The figure shows three views and two pictorial views of one solid part (mm, origin at its lowest corner). Answer the questions. Coordinates: 2 decimals unless noted, no trailing zeros. Write each loop counter-clockwise with the first axis right and the second up, starting at its lowest first coordinate (ties: lowest second). Pieces come first, ordered by that corner, then holes. Notation, with made-up numbers: M 65,36.5 L 117,36.5 A4 ccw 117,40.5 Z; hole C 63,53 d10. An arc over 180 degrees is marked long. Use a Markdown table: item, result. Add a question column.
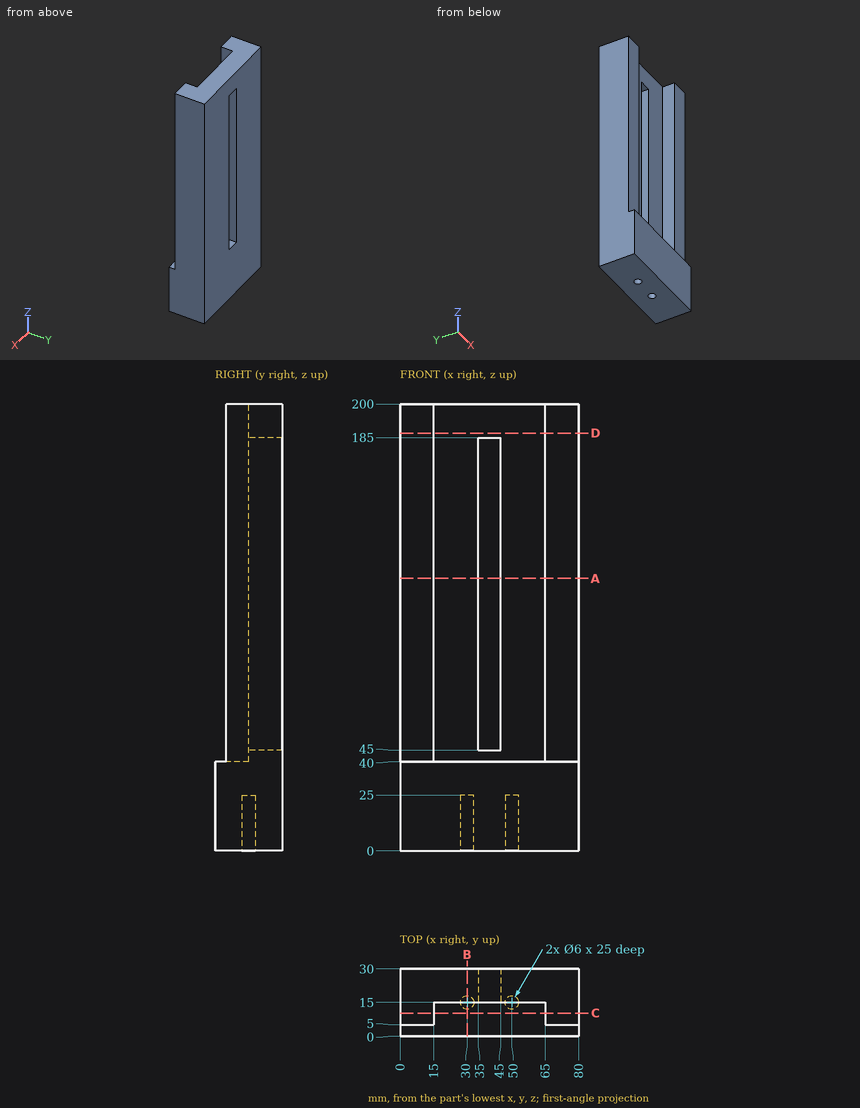
Item 1: Find section A-A on z = 122. Give the vertices of the cut face in (x, y), then the cut area to 3 significant figures.
Item 2: Find section B-B on x = 30. Give the vertices of the cut face in (y, z).
Item 3: Find section D-D on z = 187. Give the vertices of the cut face in (x, y).
Item 4: Consider probe 1 along X at (y, z) = (15, 10.5); probe 2 along Y at (x, z) = (50, 5.5); probe 3 along X at (y, z) = (27.25, 154.5). Determine where each line is inside the solid, lowest interval first.
Item 5: Find section C-C on y = 10.25. Give the vertices of the cut face in (x, z).
Item 6: Each of these flat-tipped pins is pushed along its axis until it touches: pin 1 (7.5 mm diameter, centred on x = 59, y = 10, fed in from +Z); pin 2 (8 mm diameter, centred on x = 46, z = 172.5, fed in from -Y); pin 3 (3 mm diameter, centred on x = 11.5, z = 142.5, fed in from -Y). Where does it stop, or does it pass through?
Geometry says:
| question | item | result |
|---|---|---|
| 1 | outline | M 0,5 L 15,5 L 15,15 L 35,15 L 35,30 L 0,30 Z; M 45,15 L 65,15 L 65,5 L 80,5 L 80,30 L 45,30 Z |
| 1 | area | 1,350 mm2 |
| 2 | outline | M 0,0 L 12,0 L 12,25 L 18,25 L 18,0 L 30,0 L 30,200 L 15,200 L 15,40 L 0,40 Z |
| 3 | outline | M 0,5 L 15,5 L 15,15 L 65,15 L 65,5 L 80,5 L 80,30 L 0,30 Z |
| 4 | probe 1 | x = 0 to 27, 33 to 47, 53 to 80 |
| 4 | probe 2 | y = 0 to 12, 18 to 30 |
| 4 | probe 3 | x = 0 to 35, 45 to 80 |
| 5 | outline | M 0,0 L 80,0 L 80,200 L 65,200 L 65,40 L 15,40 L 15,200 L 0,200 Z |
| 6 | pin 1 | stops at z = 40 |
| 6 | pin 2 | stops at y = 15 |
| 6 | pin 3 | stops at y = 5 |
